from build123d import *

# Parameters (mm, degrees)
SKETCH_1_W          = 40
SKETCH_1_H          = 40
SKETCH_1_R          = 1.75
SKETCH_1_R_2        = 3.1
EXTRUDE_1_DEPTH     = 9.5
FILLET_1_R          = 2
SKETCH_2_R          = 5.25
CUT_EXTRUDE_1_DEPTH = 6.2


with BuildPart() as part:
    # 草图1 → 凸台-拉伸1 (new body)
    with BuildSketch(Plane(origin=(0, 0, 0), x_dir=(1, 0, 0), z_dir=(0, 1, 0))):
        Rectangle(SKETCH_1_W, SKETCH_1_H)
        with Locations(Location((-16, 16, 0), (0, 0, 270))):  # turned: the seam where the file's is
            Circle(SKETCH_1_R, mode=Mode.SUBTRACT)
        with Locations(Location((16, 16, 0), (0, 0, 270))):  # turned: the seam where the file's is
            Circle(SKETCH_1_R, mode=Mode.SUBTRACT)
        with Locations(Location((-16, -16, 0), (0, 0, 270))):  # turned: the seam where the file's is
            Circle(SKETCH_1_R, mode=Mode.SUBTRACT)
        with Locations(Location((16, -16, 0), (0, 0, 270))):  # turned: the seam where the file's is
            Circle(SKETCH_1_R, mode=Mode.SUBTRACT)
        with Locations(Location((-12.5, 0, 0), (0, 0, 270))):  # turned: the seam where the file's is
            Circle(SKETCH_1_R_2, mode=Mode.SUBTRACT)
        with Locations(Location((12.5, 0, 0), (0, 0, 90))):  # turned: the seam where the file's is
            Circle(SKETCH_1_R_2, mode=Mode.SUBTRACT)
        with Locations(Location((0, 12.5, 0), (0, 0, 270))):  # turned: the seam where the file's is
            Circle(SKETCH_1_R_2, mode=Mode.SUBTRACT)
        with Locations(Location((0, -12.5, 0), (0, 0, 90))):  # turned: the seam where the file's is
            Circle(SKETCH_1_R_2, mode=Mode.SUBTRACT)
    extrude(amount=EXTRUDE_1_DEPTH)

    # 圆角1
    fillet_1_edges = [part.edges().sort_by_distance(p)[0] for p in [
        (20, 4.75, 20),
        (-20, 4.75, 20),
        (-20, 4.75, -20),
        (20, 4.75, -20),
    ]]
    fillet(fillet_1_edges, radius=FILLET_1_R)

    # 草图2 → 切除-拉伸1 (cut)
    with BuildSketch(Plane(origin=(0, 9.5, 0), x_dir=(1, 0, 0), z_dir=(0, 1, 0))):
        with Locations(Location((0, 12.5, 0), (0, 0, 270))):  # turned: the seam where the file's is
            Circle(SKETCH_2_R)
        with Locations(Location((12.5, 0, 0), (0, 0, 270))):  # turned: the seam where the file's is
            Circle(SKETCH_2_R)
        with Locations(Location((0, -12.5, 0), (0, 0, 270))):  # turned: the seam where the file's is
            Circle(SKETCH_2_R)
        with Locations(Location((-12.5, 0, 0), (0, 0, 270))):  # turned: the seam where the file's is
            Circle(SKETCH_2_R)
    extrude(amount=-CUT_EXTRUDE_1_DEPTH, mode=Mode.SUBTRACT)


solid = part.part
Work out the finished part from the listing and answer in its coordinate system (mm). A direction names the side the tool comes from. Coordinates: 2 decimals unless noted, no trailing zeros. Write each loop counter-clockwise with the first axis right and the second up, starting at its lowest first coordinate (ties: lowest second). Pieces come first, ordered by that corner, then holes. Notation, with made-up numbers: M 14.5,-2 L 53.5,-2 A24 ccw 53.5,27 Z; hole C 71.25,77 d10. An arc over 180 degrees is marked long. Write item = value, one per line.
1. Flat-ended cylindrical pins translate along their axes: pin 1 (3 mm diameter, centred on x = -10.5, z = -2, fed in from +Y); pin 2 (2 mm diameter, centred on x = -16, z = 16, fed in from -Y). Find the tip coordinate at first contact, or state that the pin passes through.
Solution:
pin_1 = 3.3
pin_2 = through
2. For faces 1 (the face through (10.2, 3.3, 2.3)), 2 (the face through (17.735, 4.684, -16.228)), determine the directions among +Z, -Z, +X, -X, +Y, -Y from which every point of the face is accessible in a straight line to the end or side of a thin tool.
Solution:
face_1 = +Y
face_2 = +Y, -Y
3. The part is cut by section C-C (x = 11.5). Determine the outline of the cut face in (y, z), then the cut area to 3 significant figures.
Solution:
outline = M 0,-20 L 9.5,-20 L 9.5,-5.15 L 3.3,-5.15 L 3.3,-2.93 L 0,-2.93 Z; M 0,2.93 L 3.3,2.93 L 3.3,5.15 L 9.5,5.15 L 9.5,20 L 0,20 Z
area = 297 mm2
4. Straight lines are drawn through the part: line 1 (X direction, y = 2, z = -16); line 2 (X direction, y = 5.25, z = 0); line 3 (X direction, y = 7.25, z = 12.5). For each, find the intervals that lie inside material, in ascending order. Write a range as from..to.
Solution:
line_1 = -20..-17.75, -14.25..14.25, 17.75..20
line_2 = -20..-17.75, -7.25..7.25, 17.75..20
line_3 = -20..-5.25, 5.25..20
5. The part is cut by section B-B (z = 0). Determine the outline of the cut face in (x, y), then the cut area to 3 significant figures.
Solution:
outline = M -20,0 L -15.6,0 L -15.6,3.3 L -17.75,3.3 L -17.75,9.5 L -20,9.5 Z; M -9.4,0 L 9.4,0 L 9.4,3.3 L 7.25,3.3 L 7.25,9.5 L -7.25,9.5 L -7.25,3.3 L -9.4,3.3 Z; M 15.6,0 L 20,0 L 20,9.5 L 17.75,9.5 L 17.75,3.3 L 15.6,3.3 Z
area = 209 mm2
6. Determine the mould class of faces 3 (the face through (20, 5, 0)), 4 (the face through (-0.1, 1.6, 15.6)), 5 (the face through (-19.43, 4.82, -19.4)), 6 (the face through (0.231, 6.443, 7.255)) for opening direction X: released by +X, released by -X, zero draft, split by the parting line, or undercut.
Solution:
face_3 = released by +X
face_4 = undercut
face_5 = released by -X
face_6 = undercut
7. The part is cut by section D-D (z = -12.5). Determine the outline of the cut face in (x, y).
Solution:
outline = M -20,0 L -3.1,0 L -3.1,3.3 L -5.25,3.3 L -5.25,9.5 L -20,9.5 Z; M 3.1,0 L 20,0 L 20,9.5 L 5.25,9.5 L 5.25,3.3 L 3.1,3.3 Z
8. The part is cut by section A-A (y = 7.5). State how many separate pieces and enclosed holes the cut face has, then the cut area to 3 significant figures.
Solution:
separate_pieces = 1
enclosed_holes = 8
area = 1,210 mm2
